Verification items for the finished model (mm, model axes). A direction names the side the tool comes from. Coordinates: 2 decimals unless noted, no trailing zeros. Write each loop counter-clockwise with the first axis right and the second up, starting at its lowest first coordinate (ties: lowest second). Pieces come first, ordered by that corner, then holes. Notation, with made-up numbers: (3, 16) -> (28, 16) arc R25 cw to (28, 28) -> close; hole circle Ø7 at (38, 20). An arc over 180 degrees is marked (long way). Write item = value, one per line. Start each with the question number.
(1) Section check A-A (z = -28.2). Record the cut outline in (x, y) (3 decimals).
(2) Gauge pin test, flat ends, axial feed: pin 1 Ø6 at (x, z) = (51.77, -51.77) entering from +Y; pin 2 Ø10 at (x, z) = (38.5, -47) entering from +Y; pin 3 Ø6 at (x, y) = (10.5, 16) entering from +Z; pin 4 Ø3 at (x, z) = (4.63, -51.77) entering from +Y. Record the tip position at first contact, or that the pin passes through.
(3) Section check B-B (x = 28.2). Record the cut outline in (y, z) (3 decimals).
(4) Section check D-D (x = 18). Record the cut outline in (y, z).
(5) Material ranges on probe 1 along X at (y, z) = (50.5, -4.63); probe 2 along Z at (x, y) = (51, 51); probe 3 along X at (y, z) = (50, -4), recorded low to high. Write a range as [from, to].
(6) Set-up check for faces 5 (the face through (0.48, 24.16, -42.63)), 6 (the face through (47.152, 24.157, -9.419)), 7 (the face through (9.419, 24.157, -9.248)): record each of +Z, -Z, +X, -X, +Y, -Y from which the full face is reachable in a straight line by a thin tool's end or side.
(7) Mould release check, pull along X, two halves, no side actions. Record for faces 1 (the face through (28, 27, -56.4)), 2 (the face through (52.92, 51.54, -49.55)), 3 (the face through (42.665, 24.157, -0.509)), 4 (the face through (4.09, 51.54, -49.33)): released by +X, released by -X, zero draft, split by the parting line, or undercut.
(8) Section check C-C (y = 9). Record the cut outline in (x, z), plus the area to 3 significant figures.
```python
from build123d import *

# Parameters (mm, degrees)
BOSS_EXTRUDE1_DEPTH = 54
SKETCH2_R           = 2.5
CUT_EXTRUDE1_DEPTH  = 54
SKETCH3_OUTSIDE_W   = 77.664
SKETCH3_OUTSIDE_H   = 77.664
CUT_EXTRUDE3_DEPTH  = 49
SKETCH4_R           = 19.05
BOSS_EXTRUDE2_DEPTH = 1.6
SKETCH5_R           = 3.175
BOSS_EXTRUDE3_DEPTH = 21.5


with BuildPart() as part:
    # Sketch1 → Boss-Extrude1 (new body)
    with BuildSketch(Plane(origin=(0, 0, 0), x_dir=(1, 0, 0), z_dir=(0, 1, 0))):
        with BuildLine():
            Line((0, 51.77), (0, 4.63))
            ThreePointArc((0, 4.63), (1.356095603, 1.356095603), (4.63, 0))
            Line((4.63, 0), (51.77, 0))
            ThreePointArc((51.77, 0), (55.043904397, 1.356095603), (56.4, 4.63))
            Line((56.4, 4.63), (56.4, 51.77))
            ThreePointArc((56.4, 51.77), (55.043904397, 55.043904397), (51.77, 56.4))
            Line((51.77, 56.4), (4.63, 56.4))
            ThreePointArc((4.63, 56.4), (1.356095603, 55.043904397), (0, 51.77))
        make_face()
    extrude(amount=BOSS_EXTRUDE1_DEPTH)

    # Sketch2 → Cut-Extrude1 (cut)
    with BuildSketch(Plane(origin=(0, 54, 0), x_dir=(1, 0, 0), z_dir=(0, 1, 0))):
        with Locations((4.63, 51.77)):
            Circle(SKETCH2_R)
        with Locations((51.77, 51.77)):
            Circle(SKETCH2_R)
        with Locations((51.77, 4.63)):
            Circle(SKETCH2_R)
        with Locations((4.63, 4.63)):
            Circle(SKETCH2_R)
    extrude(amount=-CUT_EXTRUDE1_DEPTH, mode=Mode.SUBTRACT)

    # Sketch3 outside → Cut-Extrude3 (cut)
    with BuildSketch(Plane.XZ):
        with Locations((28.2, -28.2)):
            Rectangle(SKETCH3_OUTSIDE_W, SKETCH3_OUTSIDE_H)
        with BuildLine():
            Line((15.067846561, -56.4), (41.332153439, -56.4))
            ThreePointArc((41.332153439, -56.4), (42.650046494, -55.904379571), (43.314764828, -54.663157895))
            ThreePointArc((43.314764828, -54.663157895), (47.066190488, -47.066190488), (54.663157895, -43.314764828))
            ThreePointArc((54.663157895, -43.314764828), (55.904379571, -42.650046494), (56.4, -41.332153439))
            Line((56.4, -41.332153439), (56.4, -15.067846561))
            ThreePointArc((56.4, -15.067846561), (55.904379571, -13.749953506), (54.663157895, -13.085235172))
            ThreePointArc((54.663157895, -13.085235172), (47.066190488, -9.333809512), (43.314764828, -1.736842105))
            ThreePointArc((43.314764828, -1.736842105), (42.650046494, -0.495620429), (41.332153439, 0))
            Line((41.332153439, 0), (15.067846561, 0))
            ThreePointArc((15.067846561, 0), (13.749953506, -0.495620429), (13.085235172, -1.736842105))
            ThreePointArc((13.085235172, -1.736842105), (9.333809512, -9.333809512), (1.736842105, -13.085235172))
            ThreePointArc((1.736842105, -13.085235172), (0.495620429, -13.749953506), (0, -15.067846561))
            Line((0, -15.067846561), (0, -41.332153439))
            ThreePointArc((0, -41.332153439), (0.495620429, -42.650046494), (1.736842105, -43.314764828))
            ThreePointArc((1.736842105, -43.314764828), (9.333809512, -47.066190488), (13.085235172, -54.663157895))
            ThreePointArc((13.085235172, -54.663157895), (13.749953506, -55.904379571), (15.067846561, -56.4))
        make_face(mode=Mode.SUBTRACT)
    extrude(amount=-CUT_EXTRUDE3_DEPTH, mode=Mode.SUBTRACT)

    # Sketch4 → Boss-Extrude2 (add)
    with BuildSketch(Plane(origin=(0, 54, 0), x_dir=(1, 0, 0), z_dir=(0, 1, 0))):
        with Locations((28.2, 28.2)):
            Circle(SKETCH4_R)
    extrude(amount=BOSS_EXTRUDE2_DEPTH)

    # Sketch5 → Boss-Extrude3 (add)
    with BuildSketch(Plane(origin=(0, 55.6, 0), x_dir=(1, 0, 0), z_dir=(0, 1, 0))):
        with Locations((28.2, 28.2)):
            Circle(SKETCH5_R)
    extrude(amount=BOSS_EXTRUDE3_DEPTH)


solid = part.part
```
Response:
q1.outline = (0, 0) -> (56.4, 0) -> (56.4, 54) -> (47.25, 54) -> (47.25, 55.6) -> (31.375, 55.6) -> (31.375, 77.1) -> (25.025, 77.1) -> (25.025, 55.6) -> (9.15, 55.6) -> (9.15, 54) -> (0, 54) -> close
q2.pin_1 = 54
q2.pin_2 = 55.6
q2.pin_3 = -0.76
q2.pin_4 = through
q3.outline = (0, -56.4) -> (54, -56.4) -> (54, -47.25) -> (55.6, -47.25) -> (55.6, -31.375) -> (77.1, -31.375) -> (77.1, -25.025) -> (55.6, -25.025) -> (55.6, -9.15) -> (54, -9.15) -> (54, 0) -> (0, 0) -> close
q4.outline = (0, -56.4) -> (54, -56.4) -> (54, -44.29) -> (55.6, -44.29) -> (55.6, -12.11) -> (54, -12.11) -> (54, 0) -> (0, 0) -> close
q5.probe_1 = [0, 2.13], [7.13, 49.27], [54.27, 56.4]
q5.probe_2 = [-56.4, -54.15], [-49.39, -7.01], [-2.25, 0]
q5.probe_3 = [0.04, 2.21], [7.05, 49.35], [54.19, 56.36]
q6.face_5 = -Z, -X, -Y
q6.face_6 = +Z, +X, -Y
q6.face_7 = +Z, -X, -Y
q7.face_1 = zero draft
q7.face_2 = undercut
q7.face_3 = released by +X
q7.face_4 = undercut
q8.outline = (0, -41.33) arc R2 ccw to (1.74, -43.31) arc R13.2 cw to (13.09, -54.66) arc R2 ccw to (15.07, -56.4) -> (41.33, -56.4) arc R2 ccw to (43.31, -54.66) arc R13.2 cw to (54.66, -43.31) arc R2 ccw to (56.4, -41.33) -> (56.4, -15.07) arc R2 ccw to (54.66, -13.09) arc R13.2 cw to (43.31, -1.74) arc R2 ccw to (41.33, 0) -> (15.07, 0) arc R2 ccw to (13.09, -1.74) arc R13.2 cw to (1.74, -13.09) arc R2 ccw to (0, -15.07) -> close
q8.area = 2,630 mm2
